Build history of the part. All positions in model axes, mm. Round coordinates to 2 decimals unless told otherwise and drop trailing zeros. Write each loop counter-clockwise with the first axis right and the second up, starting at its lowest first coordinate (ties: lowest second). Pieces come first, ordered by that corner, then holes. Notation, with made-up numbers: (-12, 12) -> (19, 12) arc R13 ccw to (19, 32) -> close; hole circle Ø6 at (-40, -29). An arc over 180 degrees is marked (long way). Answer in a Markdown table with one row per item.
```python
from build123d import *

# Parameters (mm, degrees)
F0_W     = 120.127284
F0_H     = 9.181094
F0_W_2   = 25
F0_H_2   = 5
F1_DEPTH = 6.35
F2_R     = 1


with BuildPart() as f1:
    # F0 (on Top) → F1 (new body)
    with BuildSketch(Plane.XY):
        Rectangle(F0_W, F0_H)
        with Locations((-45.202259, 0)):
            Rectangle(F0_W_2, F0_H_2, mode=Mode.SUBTRACT)
        with Locations((45.202259, 0)):
            Rectangle(F0_W_2, F0_H_2, mode=Mode.SUBTRACT)
    extrude(amount=F1_DEPTH)

    # F2
    f2_edges = [f1.edges().sort_by_distance(p)[0] for p in [
        (-57.702259, 2.5, 3.175),
        (-57.702259, -2.5, 3.175),
        (57.702259, 2.5, 3.175),
        (57.702259, -2.5, 3.175),
        (32.702259, -2.5, 3.175),
        (32.702259, 2.5, 3.175),
        (-32.702259, -2.5, 3.175),
        (-32.702259, 2.5, 3.175),
    ]]
    fillet(f2_edges, radius=F2_R)


solid = f1.part
```
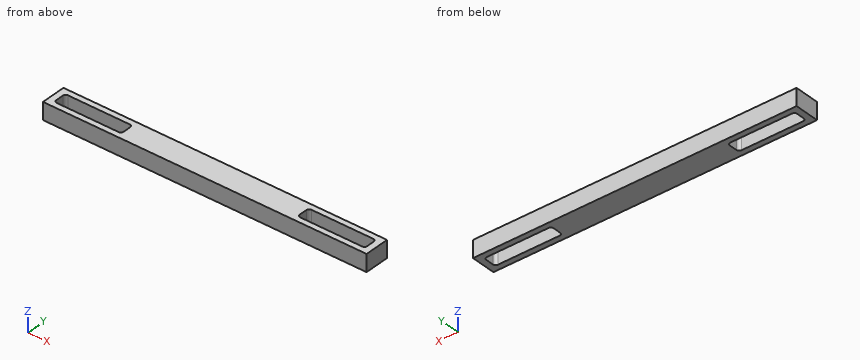
Q1. Saw through at B-B on z = 1. Write the cut outline in (x, y).
A:
| item | result |
|---|---|
| outline | (-60.06, -4.59) -> (60.06, -4.59) -> (60.06, 4.59) -> (-60.06, 4.59) -> close; hole (-57.7, -1.5) arc R1 ccw to (-56.7, -2.5) -> (-33.7, -2.5) arc R1 ccw to (-32.7, -1.5) -> (-32.7, 1.5) arc R1 ccw to (-33.7, 2.5) -> (-56.7, 2.5) arc R1 ccw to (-57.7, 1.5) -> close; hole (32.7, -1.5) arc R1 ccw to (33.7, -2.5) -> (56.7, -2.5) arc R1 ccw to (57.7, -1.5) -> (57.7, 1.5) arc R1 ccw to (56.7, 2.5) -> (33.7, 2.5) arc R1 ccw to (32.7, 1.5) -> close |
Q2. Saw through at C-C on y = 0.5. Write the cut outline in (x, z), plus the area to 3 significant figures.
A:
| item | result |
|---|---|
| outline | (-60.06, 0) -> (-57.7, 0) -> (-57.7, 6.35) -> (-60.06, 6.35) -> close; (-32.7, 0) -> (32.7, 0) -> (32.7, 6.35) -> (-32.7, 6.35) -> close; (57.7, 0) -> (60.06, 0) -> (60.06, 6.35) -> (57.7, 6.35) -> close |
| area | 445 mm² |
Q3. Wall check: line 1 (X direction, y = 0.5, z = 2.75); line 2 (Y direction, x = -44, z = 5.5); line 3 (X direction, y = -2, z = 5). Give the ranges that are in metal, low to high. Write a range as [from, to].
A:
| item | result |
|---|---|
| line 1 | [-60.06, -57.7], [-32.7, 32.7], [57.7, 60.06] |
| line 2 | [-4.59, -2.5], [2.5, 4.59] |
| line 3 | [-60.06, -57.57], [-32.84, 32.84], [57.57, 60.06] |
Q4. Saw through at A-A on x = -51.5. Write the cut outline in (y, z), plus the area to 4 significant figures.
A:
| item | result |
|---|---|
| outline | (-4.59, 0) -> (-2.5, 0) -> (-2.5, 6.35) -> (-4.59, 6.35) -> close; (2.5, 0) -> (4.59, 0) -> (4.59, 6.35) -> (2.5, 6.35) -> close |
| area | 26.55 mm² |
